Drawing for the job (mm, zero at the part's lowest x, y, z). Round coordinates to 2 decimals unless told otherwise and drop trailing zeros. Loops run counter-clockwise (first coordinate to the right, second up) from the corner with the lowest first, then second, coordinate; pieces in that order, holes last. Notation, with made-up numbers: (48.5, 40.5) - (70.5, 40.5) arc R38 cw to (70.5, 78.5) - close; hole circle Ø8 at (-25.75, 7.5). An arc over 180 degrees is marked (long way). Put each result on its own line as item: value.
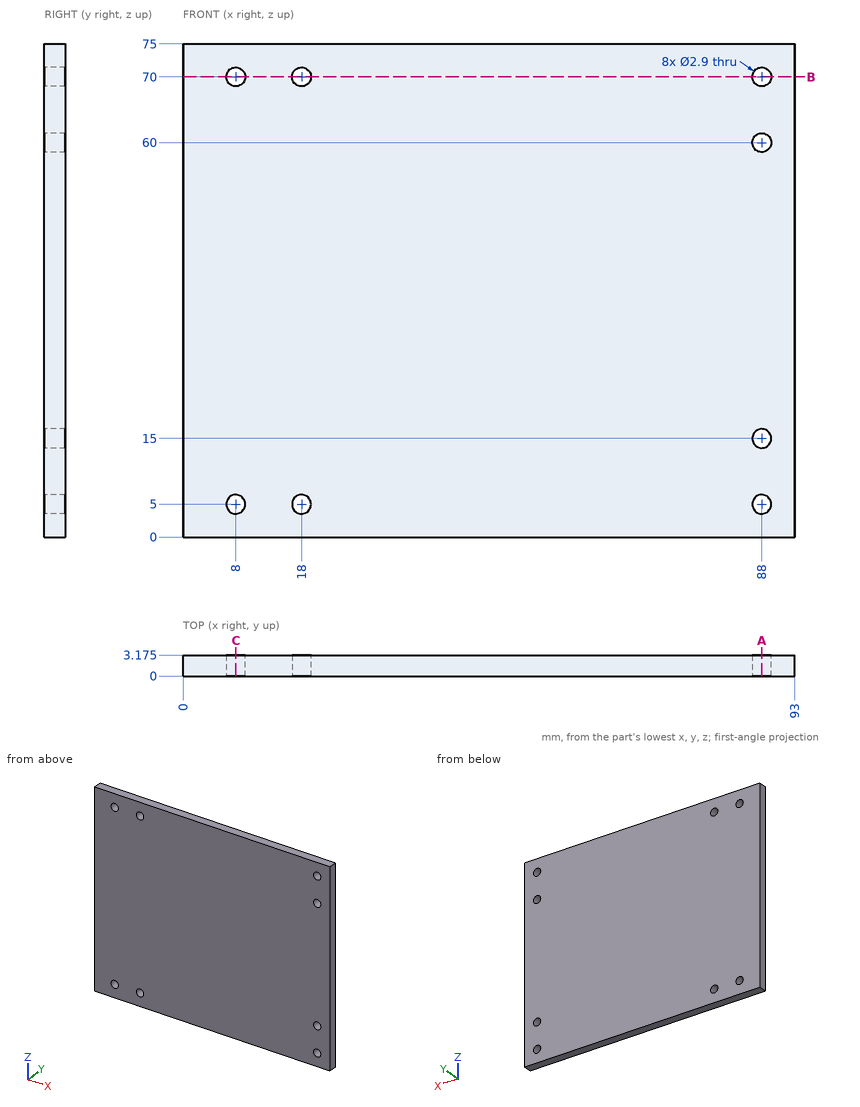
1. Band-saw the part on B-B (z = 70). List the corners of the cut face in (x, y) (3 decimals), plus the area to 3 significant figures.
A:
outline: (0, 0) - (6.55, 0) - (6.55, 3.175) - (0, 3.175) - close; (9.45, 0) - (16.55, 0) - (16.55, 3.175) - (9.45, 3.175) - close; (19.45, 0) - (86.55, 0) - (86.55, 3.175) - (19.45, 3.175) - close; (89.45, 0) - (93, 0) - (93, 3.175) - (89.45, 3.175) - close
area: 268 mm²
2. Band-saw the part on C-C (x = 8). List the corners of the cut face in (y, z) (3 decimals), plus the area to 3 significant figures.
A:
outline: (0, 0) - (3.175, 0) - (3.175, 3.55) - (0, 3.55) - close; (0, 6.45) - (3.175, 6.45) - (3.175, 68.55) - (0, 68.55) - close; (0, 71.45) - (3.175, 71.45) - (3.175, 75) - (0, 75) - close
area: 220 mm²
3. Pin check, flat tip, straight feed: P1, Ø2.5, axis at x = 18, z = 5, coming from the -Y side. Stop position of the tip, or through.
A:
P1: passes through
4. Band-saw the part on A-A (x = 88). List the corners of the cut face in (y, z) (3 decimals).
A:
outline: (0, 0) - (3.175, 0) - (3.175, 3.55) - (0, 3.55) - close; (0, 6.45) - (3.175, 6.45) - (3.175, 13.55) - (0, 13.55) - close; (0, 16.45) - (3.175, 16.45) - (3.175, 58.55) - (0, 58.55) - close; (0, 61.45) - (3.175, 61.45) - (3.175, 68.55) - (0, 68.55) - close; (0, 71.45) - (3.175, 71.45) - (3.175, 75) - (0, 75) - close
5. Probe line 1 along Z through (x, y) = (88, 2.2); line 2 along Z through (x, y) = (18, 1.2); line 3 along X through (y, z) = (0.75, 70). List the from-to ranges inside material, lowest first. Write a range as [from, to].
A:
line 1: z = [0, 3.55], [6.45, 13.55], [16.45, 58.55], [61.45, 68.55], [71.45, 75]
line 2: z = [0, 3.55], [6.45, 68.55], [71.45, 75]
line 3: x = [0, 6.55], [9.45, 16.55], [19.45, 86.55], [89.45, 93]
